Work out the finished part from the listing and answer in its coordinate system (mm). Face numbers are marked on the shaded views. Give positions to 0.01 mm unless a question says otherwise; leave off trailing zeros. Loops run counter-clockwise (first coordinate to the right, second up) from the corner with the lowest first, then second, coordinate; pieces in that order, holes last. Notation, with made-up numbers: (45, -1.75) - (50, -1.75) arc R18 cw to (50, 12.25) - close; hole circle Ø10 at (82.5, -15). An arc over 180 degrees is marked (long way). One line per question, with ' | ' between items.
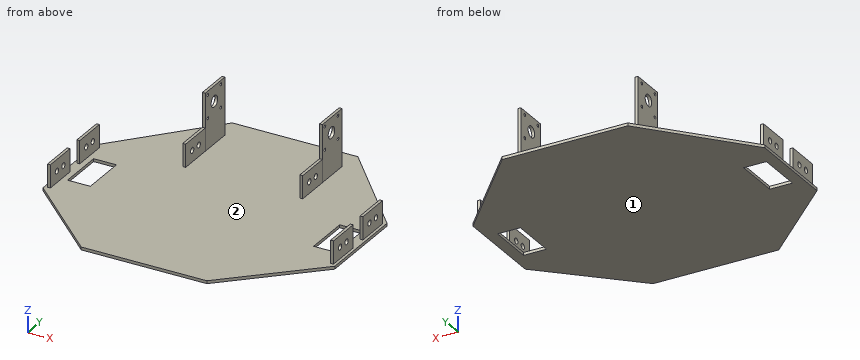
from build123d import *

# Parameters (mm, degrees)
F1_DEPTH  = 3.175
F2_W      = 3.175
F2_H      = 38.1
F3_DEPTH  = 25.4
F4_R      = 3.175
F5_DEPTH  = 381
F2_W_2    = 25.4
F2_H_2    = 50.8
F6_DEPTH  = 25.4
F7_DEPTH  = 63.5
F8_R      = 6.35
F9_DEPTH  = 177.8
F11_DEPTH = 304.8
F12_DEPTH = 25.4
F13_DEPTH = 254


# Not quite as in the source:
# - ends of sketch curves that miss each other by under 0.0002 mm in the source are joined
# - a feature names something its author has since deleted; it is built from what else it names


with BuildPart() as f1:
    # F0 (on Top) → F1 (new body)
    with BuildSketch(Plane.XY):
        Polygon((-252.9524413709, 74.0429753427), (-252.9524413709, -27.5570246573), (-160.6017448068, -114.7370042634), (-20.9017448068, -114.7370042634), (71.4489517573, -27.5570246573), (71.4489517573, 74.0429753427), (-20.9017448068, 178.8639600935), (-160.6017448068, 178.8639600935), align=None)
    extrude(amount=F1_DEPTH)

    # F2 (on face) → F3 (join)
    with BuildSketch(Plane.XY.offset(3.175)):
        with Locations((-248.1899413709, 51.8179753427)):
            Rectangle(F2_W, F2_H)
        with Locations((-248.1899413709, -5.3320246573)):
            Rectangle(F2_W, F2_H)
        with Locations((-155.8392448068, 96.3139587522)):
            Rectangle(F2_W, F2_H)
        with Locations((-25.6642448068, 96.3139587522)):
            Rectangle(F2_W, F2_H)
        with Locations((66.6864517573, 51.8179753427)):
            Rectangle(F2_W, F2_H)
        with Locations((66.6864517573, -5.3320246573)):
            Rectangle(F2_W, F2_H)
    extrude(amount=F3_DEPTH)

    # F4 (on Right) → F5 (cut, symmetric)
    with BuildSketch(Plane.YZ):
        with Locations((-11.6820246573, 15.875)):
            Circle(F4_R)
        with Locations((1.0179753427, 15.875)):
            Circle(F4_R)
        with Locations((45.4679753427, 15.875)):
            Circle(F4_R)
        with Locations((58.1679753427, 15.875)):
            Circle(F4_R)
        with Locations((89.9639587522, 15.875)):
            Circle(F4_R)
        with Locations((102.6639587522, 15.875)):
            Circle(F4_R)
    extrude(amount=F5_DEPTH, both=True, mode=Mode.SUBTRACT)

    # F2 (on face) → F6 (cut)
    with BuildSketch(Plane.XY.offset(3.175)):
        with Locations((-227.5524413709, 23.2429753427)):
            Rectangle(F2_W_2, F2_H_2)
        with Locations((46.0489517573, 23.2429753427)):
            Rectangle(F2_W_2, F2_H_2)
    extrude(amount=-F6_DEPTH, mode=Mode.SUBTRACT)

    # F2 (on face) → F7 (join)
    with BuildSketch(Plane.XY.offset(3.175)):
        with Locations((-155.8392446995, 134.4139587522)):
            Rectangle(F2_W, F2_H)
        with Locations((-25.6642446429, 134.4139587522)):
            Rectangle(F2_W, F2_H)
    extrude(amount=F7_DEPTH)

    # F8 (on face) + F4 (on Right) → F9 (cut, symmetric)
    with BuildSketch(Plane.YZ.offset(-24.0767446429)):
        with Locations((133.1326216459, 49.6721826494)):
            Circle(F8_R)
    with BuildSketch(Plane.YZ):
        with Locations((89.9639587522, 15.875)):
            Circle(F4_R)
        with Locations((102.6639587522, 15.875)):
            Circle(F4_R)
    extrude(amount=F9_DEPTH, both=True, mode=Mode.SUBTRACT)

    # F10 (on face) → F11 (cut)
    with BuildSketch(Plane.YZ.offset(-24.0767446429)):
        with BuildLine():
            ThreePointArc((122.0201216459, 62.3721826494), (119.3100896308, 63.4947146645), (120.4326216459, 60.7846826494))
            Line((120.4326216459, 60.7846826494), (120.4326216459, 62.3721826494))
            Line((120.4326216459, 62.3721826494), (122.0201216459, 62.3721826494))
        make_face()
        with BuildLine():
            Line((145.8326216459, 62.3721826494), (145.8326216459, 60.7846826494))
            ThreePointArc((145.8326216459, 60.7846826494), (146.9551536611, 61.2496506342), (147.4201216459, 62.3721826494))
            ThreePointArc((147.4201216459, 62.3721826494), (145.8326216459, 63.9596826494), (144.2451216459, 62.3721826494))
            Line((144.2451216459, 62.3721826494), (145.8326216459, 62.3721826494))
        make_face()
        with BuildLine():
            Line((145.8326216459, 36.9721826494), (144.2451216459, 36.9721826494))
            ThreePointArc((144.2451216459, 36.9721826494), (145.8326216459, 35.3846826494), (147.4201216459, 36.9721826494))
            ThreePointArc((147.4201216459, 36.9721826494), (146.9551536611, 38.0947146645), (145.8326216459, 38.5596826494))
            Line((145.8326216459, 38.5596826494), (145.8326216459, 36.9721826494))
        make_face()
        with BuildLine():
            ThreePointArc((120.4326216459, 38.5596826494), (119.3100896308, 35.8496506342), (122.0201216459, 36.9721826494))
            Line((122.0201216459, 36.9721826494), (120.4326216459, 36.9721826494))
            Line((120.4326216459, 36.9721826494), (120.4326216459, 38.5596826494))
        make_face()
        with BuildLine():
            Line((120.4326216459, 36.9721826494), (122.0201216459, 36.9721826494))
            ThreePointArc((122.0201216459, 36.9721826494), (121.5551536611, 38.0947146645), (120.4326216459, 38.5596826494))
            Line((120.4326216459, 38.5596826494), (120.4326216459, 36.9721826494))
        make_face()
        with BuildLine():
            Line((120.4326216459, 62.3721826494), (120.4326216459, 60.7846826494))
            ThreePointArc((120.4326216459, 60.7846826494), (121.5551536611, 61.2496506342), (122.0201216459, 62.3721826494))
            Line((122.0201216459, 62.3721826494), (120.4326216459, 62.3721826494))
        make_face()
        with BuildLine():
            ThreePointArc((144.2451216459, 62.3721826494), (144.7100896308, 61.2496506342), (145.8326216459, 60.7846826494))
            Line((145.8326216459, 60.7846826494), (145.8326216459, 62.3721826494))
            Line((145.8326216459, 62.3721826494), (144.2451216459, 62.3721826494))
        make_face()
        with BuildLine():
            ThreePointArc((145.8326216459, 38.5596826494), (144.7100896308, 38.0947146645), (144.2451216459, 36.9721826494))
            Line((144.2451216459, 36.9721826494), (145.8326216459, 36.9721826494))
            Line((145.8326216459, 36.9721826494), (145.8326216459, 38.5596826494))
        make_face()
    extrude(amount=-F11_DEPTH, mode=Mode.SUBTRACT)

    # F2 (on face) → F12 (join)
    with BuildSketch(Plane.XY.offset(3.175)):
        with Locations((-25.6642448068, 96.3139587522)):
            Rectangle(F2_W, F2_H)
        with Locations((-155.8392448068, 96.3139587522)):
            Rectangle(F2_W, F2_H)
    extrude(amount=F12_DEPTH)

    # F4 (on Right) → F13 (cut)
    with BuildSketch(Plane.YZ):
        with Locations((102.6639587522, 15.875)):
            Circle(F4_R)
        with Locations((89.9639587522, 15.875)):
            Circle(F4_R)
    extrude(amount=-F13_DEPTH, mode=Mode.SUBTRACT)


solid = f1.part
1. Consider L1, parallel to Z at x = -85.5, y = -47 (3 decimals); L2, parallel to X at y = -8, z = 17.5; L3, parallel to Y at x = -155.5, z = 29. Determine where each line is inside the solid, lowest interval first.
Evaluation:
L1: 0 to 3.175 | L2: -249.78 to -246.6, 65.1 to 68.27 | L3: 115.36 to 153.46
2. Flat-ended cylindrical pins translate along their axes: pin 1 (19 mm diameter, centred on y = 134.5, z = 25.5, fed in from -X); pin 2 (12.5 mm diameter, centred on y = -14.5, z = 21, fed in from -X); pin 3 (7.5 mm diameter, centred on y = 93.5, z = 20.5, fed in from +X). Find the tip coordinate at first contact, or state that the pin passes through.
Evaluation:
pin 1: x = -157.43 | pin 2: x = -249.78 | pin 3: x = -24.08
3. Find section C-C on y = -46.5. Write down the section's boundary in (x, z) (3 decimals), then the cut area to 3 significant figures.
Evaluation:
outline: (-232.886, 0) - (51.382, 0) - (51.382, 3.175) - (-232.886, 3.175) - close | area: 903 mm2
4. Find section A-A on z = 25. Write down the section's boundary in (x, y).
Evaluation:
outline: (-249.78, -24.38) - (-246.6, -24.38) - (-246.6, 13.72) - (-249.78, 13.72) - close; (-249.78, 32.77) - (-246.6, 32.77) - (-246.6, 70.87) - (-249.78, 70.87) - close; (-157.43, 77.26) - (-154.25, 77.26) - (-154.25, 153.46) - (-157.43, 153.46) - close; (-27.25, 77.26) - (-24.08, 77.26) - (-24.08, 153.46) - (-27.25, 153.46) - close; (65.1, -24.38) - (68.27, -24.38) - (68.27, 13.72) - (65.1, 13.72) - close; (65.1, 32.77) - (68.27, 32.77) - (68.27, 70.87) - (65.1, 70.87) - close
5. Find section B-B on x = -100. Write down the section's boundary in (y, z) (3 decimals).
Evaluation:
outline: (-114.737, 0) - (178.864, 0) - (178.864, 3.175) - (-114.737, 3.175) - close
6. Determine the mould class of the marked faces 1 and 2 for opening direction X: +X half, -X half, draft (parallel to the pull), parting line (faces both ways), or undercut.
Evaluation:
face 1: draft | face 2: undercut
